Build history of the part. All positions in model axes, mm. A direction names the side the tool comes from. Give positions to 0.01 mm unless a question says otherwise; leave off trailing zeros. Loops run counter-clockwise (first coordinate to the right, second up) from the corner with the lowest first, then second, coordinate; pieces in that order, holes last. Notation, with made-up numbers: M 59,51 L 113,51 A13 cw 113,68 Z; hole C 57.5,41 d8. An arc over 180 degrees is marked long. Answer as a JSON object with one key per item and string values. Group by question number.
1. Slice it at B-B (z = 45). List the corners of the cut face in (x, y) (3 decimals), then the cut area to 3 significant figures.
2. 3-axis set-ups, long thin cutter, end or side, ignore diameter. For faces 4 (the face through (-91.44, -5, 29)), 5 (the face through (-97, -96, 0)), 6 (the face through (-5, -91.44, 29)), 7 (the face through (-53.14, -48.654, 76.378)): which of +Z, -Z, +X, -X, +Y, -Y reach the whole face in a straight line?
3. Drop flat-ended pins along their axis: pin 1 Ø6 at (x, y) = (-75.5, -48) entering from +Z; pin 2 Ø11 at (x, z) = (-96, 17.5) entering from +Y; pin 3 Ø5 at (x, y) = (-51.5, -50) entering from -Z; pin 4 Ø8 at (x, y) = (-41.5, -28) entering from -Z. Give the stop position or say it passes through.
4. Mould opens along X. For faces 1 (the face through (-97, -5, 0)), 2 (the face through (-101.6, -51, 60)), 3 (the face through (-10.16, -96, 29)) say: released by +X, released by -X, zero draft, split by the parting line, or undercut.
5. Slice it at A-A (z = 27). List the corners of the cut face in (x, y).
6. Drill centre lines: line 1 along Z through (x, y) = (-96.5, -76); line 2 along Z through (x, y) = (-6, -92.5). Where is each one in solid material? Low to high. Write a range as [from, to].
7. Slice it at C-C (x = -50.8). List the corners of the cut face in (y, z) (3 decimals).
from build123d import *

# Parameters (mm, degrees)
F0_W     = 101.6
F0_H     = 101.6
F1_DEPTH = 63.5
F2_W     = 81.28
F2_H     = 81.28
F2_W_2   = 10.16
F2_H_2   = 10.16
F3_DEPTH = 59.69
F5_DEPTH = 63.501
F6_R     = 3.175
F7_DEPTH = 25.4


with BuildPart() as f1:
    # F0 (on Top) → F1 (new body)
    with BuildSketch(Plane.XY):
        with Locations((-50.8, -50.8)):
            Rectangle(F0_W, F0_H)
    extrude(amount=F1_DEPTH)

    # F2 (on face) → F3 (cut)
    with BuildSketch(Plane(origin=(0, 0, 0), x_dir=(1, 0, 0), z_dir=(0, 0, -1))):
        with Locations((-50.8, 50.8)):
            Rectangle(F2_W, F2_H)
        with Locations((-5.08, 50.8)):
            Rectangle(F2_W_2, F2_H)
        with Locations((-50.8, 5.08)):
            Rectangle(F2_W, F2_H_2)
        with Locations((-96.52, 50.8)):
            Rectangle(F2_W_2, F2_H)
        with Locations((-50.8, 96.52)):
            Rectangle(F2_W, F2_H_2)
    extrude(amount=-F3_DEPTH, mode=Mode.SUBTRACT)

    # F4 (on face) → F5 (cut, through all)
    with BuildSketch(Plane.XY.offset(63.5)):
        with BuildLine():
            ThreePointArc((-47.625, -50.8), (-49.5849801022, -47.8666824843), (-53.0450640303, -48.5549359697))
            Line((-53.0450640303, -48.5549359697), (-48.5549359697, -53.0450640303))
            ThreePointArc((-48.5549359697, -53.0450640303), (-47.8666824843, -52.0150198978), (-47.625, -50.8))
        make_face()
        with BuildLine():
            Line((-48.5549359697, -53.0450640303), (-53.0450640303, -48.5549359697))
            ThreePointArc((-53.0450640303, -48.5549359697), (-53.0450640303, -53.0450640303), (-48.5549359697, -53.0450640303))
        make_face()
    extrude(amount=-F5_DEPTH, mode=Mode.SUBTRACT)

    # F6 (on face) → F7 (join, symmetric)
    with BuildSketch(Plane.XY.offset(63.5)):
        with Locations((-50.8, -50.8)):
            Circle(F6_R)
    extrude(amount=F7_DEPTH, both=True)


solid = f1.part
Established:
{
 "1": {"outline": "M -101.6,-101.6 L -91.44,-101.6 L -91.44,-91.44 L -101.6,-91.44 Z; M -101.6,-10.16 L -91.44,-10.16 L -91.44,0 L -101.6,0 Z; C -50.8,-50.8 d6.35; M -10.16,-101.6 L 0,-101.6 L 0,-91.44 L -10.16,-91.44 Z; M -10.16,-10.16 L 0,-10.16 L 0,0 L -10.16,0 Z", "area": "445 mm^2"},
 "2": {"face 4": "-Z, +Y, -Y", "face 5": "-Z, +X, -X, +Y, -Y", "face 6": "-Z, +X, -X", "face 7": "+Z"},
 "3": {"pin 1": "stops at z = 63.5", "pin 2": "stops at y = 0", "pin 3": "stops at z = 38.1", "pin 4": "stops at z = 59.69"},
 "4": {"face 1": "zero draft", "face 2": "released by -X", "face 3": "undercut"},
 "5": {"outline": "M -101.6,-101.6 L -91.44,-101.6 L -91.44,-91.44 L -101.6,-91.44 Z; M -101.6,-10.16 L -91.44,-10.16 L -91.44,0 L -101.6,0 Z; M -10.16,-101.6 L 0,-101.6 L 0,-91.44 L -10.16,-91.44 Z; M -10.16,-10.16 L 0,-10.16 L 0,0 L -10.16,0 Z"},
 "6": {"line 1": "z = [59.69, 63.5]", "line 2": "z = [0, 63.5]"},
 "7": {"outline": "M -101.6,59.69 L -53.975,59.69 L -53.975,38.1 L -47.625,38.1 L -47.625,59.69 L 0,59.69 L 0,63.5 L -47.625,63.5 L -47.625,88.9 L -53.975,88.9 L -53.975,63.5 L -101.6,63.5 Z"}
}
